Can you work these out from the model? Positions are in its coordinate system, mm. A direction names the side the tool comes from. Give positions to 0.01 mm unless a question says otherwise; leave off trailing zeros. Loops run counter-clockwise (first coordinate to the right, second up) from the corner with the lowest first, then second, coordinate; pieces in that order, holes last. Notation, with made-up numbers: (26.5, 6.25) - (85.5, 6.25) arc R29 cw to (85.5, 40.25) - close; hole circle Ø3 at (-10, 14.25). An arc over 180 degrees is marked (long way). Write item = value, one per line.
from build123d import *

# Parameters (mm, degrees)
CORTAR_EXTRUIR2_DEPTH = 1
CHAFL_N1_SIZE         = 0.2


with BuildPart() as part:
    # Croquis1 → Revolución1 (revolve)
    with BuildSketch(Plane(origin=(0, 0, 0), x_dir=(0, 0, -1), z_dir=(1, 0, 0)), mode=Mode.PRIVATE) as revoluci_n1_sk:
        with BuildLine():
            Line((0, 3), (0, 1.5))
            Line((0, 1.5), (8, 1.5))
            Line((8, 1.5), (8, 0))
            Line((8, 0), (-2.4, 0))
            Line((-2.4, 0), (-2.4, 0.438750305))
            ThreePointArc((-2.4, 0.438750305), (-1.967126393, 1.948717192), (-0.8, 3))
            Line((-0.8, 3), (0, 3))
        make_face()
    revolve(revoluci_n1_sk.sketch.rotate(Axis((0, 0, -8), (0, 0, -1)), 180), axis=Axis((0, 0, -8), (0, 0, -1)))

    # Croquis2 → Cortar-Extruir2 (cut)
    with BuildSketch(Plane.XY.offset(2.4)):
        Polygon((-0.35, 0.35), (-1.75, 0.35), (-1.75, -0.35), (-0.35, -0.35), (-0.35, -1.75), (0.35, -1.75), (0.35, -0.35), (1.75, -0.35), (1.75, 0.35), (0.35, 0.35), (0.35, 1.75), (-0.35, 1.75), align=None)
    extrude(amount=-CORTAR_EXTRUIR2_DEPTH, mode=Mode.SUBTRACT)

    # Chaflán1
    chafl_n1_edges = [part.edges().sort_by_distance(p)[0] for p in [
        (0, 1.5, -8),
    ]]
    chamfer(chafl_n1_edges, length=CHAFL_N1_SIZE)


solid = part.part
Q1. We'd pull the mould along Y, two halves only. Please class faces 3 (the cylindrical face through (-0.45, -1.43, -3.95)), 4 (the flat face through (1.3, -1.3, 0)), 5 (the flat face through (1, 0.35, 2)): released by +Y, released by -Y, zero draft, split by the parting line, or undercut.
Output:
face_3 = split by the parting line
face_4 = zero draft
face_5 = undercut
Q2. Imagine slicing it at A-A, the plane z = -4.5. Write out the boundary of the cut face in (x, y).
Output:
outline = circle Ø3 at (0, 0)
Q3. For pin 1 (0.5 mm diameter, centred on y = -1.5, z = 2, fed in from -X); pin 2 (0.5 mm diameter, centred on y = 0.5, z = 2, fed in from +X); pin 3 (0.8 mm diameter, centred on y = 1.5, z = 2, fed in from -X), each with a flat end and sliding along its axis, tell me the tip position at first contact or that it passes through.
Output:
pin_1 = -1.73
pin_2 = 2.2
pin_3 = -1.97
Q4. I need wall thicknesses on L1, parallel to X at y = -0.75, z = -6.25; L2, parallel to Y at x = -1.25, z = 1.75; L3, parallel to Z at x = 0.75, y = -2.5. Which ranges of each line are inside material? Lowest first, please.
Output:
L1 = -1.3 to 1.3
L2 = -1.87 to -0.35, 0.35 to 1.87
L3 = 0 to 1.4
Q5. Which directions (+Z, -Z, +X, -X, +Y, -Y) give clear straight access to the entire face, cutting with the end or side of a thin tool? Please do faces 1 (the flat face through (-1, 0.35, 2)), 2 (the cylindrical face through (-0.9, -2.86, 0.39)).
Output:
face_1 = +Z
face_2 = +Z, -Z
